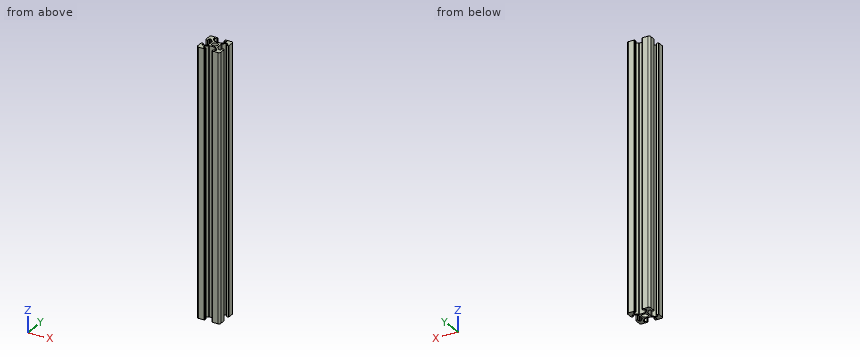
```python
from build123d import *

# Parameters (mm, degrees)
SKETCH_1_R      = 2.5
EXTRUDE_1_DEPTH = 230
FILLET_1_R      = 1.5


with BuildPart() as part:
    # 草图1 → 凸台-拉伸1 (new body)
    with BuildSketch(Plane.XY):
        with BuildLine():
            Line((20, 13.6), (20, 20))
            Line((20, 20), (13.6, 20))
            Line((13.6, 20), (13.6, 19.8))
            Line((13.6, 19.8), (13.2, 19.8))
            ThreePointArc((13.2, 19.8), (13.129289322, 19.770710678), (13.1, 19.7))
            Line((13.1, 19.7), (13.1, 18.3))
            ThreePointArc((13.1, 18.3), (13.129289322, 18.229289322), (13.2, 18.2))
            Line((13.2, 18.2), (15.2, 18.2))
            ThreePointArc((15.2, 18.2), (15.412132034, 18.112132034), (15.5, 17.9))
            Line((15.5, 17.9), (15.5, 16.974873734))
            ThreePointArc((15.5, 16.974873734), (15.423879533, 16.592190302), (15.207106781, 16.267766953))
            Line((15.207106781, 16.267766953), (13.132233047, 14.192893219))
            ThreePointArc((13.132233047, 14.192893219), (12.807809698, 13.976120467), (12.425126266, 13.9))
            Line((12.425126266, 13.9), (7.574873734, 13.9))
            ThreePointArc((7.574873734, 13.9), (7.192190302, 13.976120467), (6.867766953, 14.192893219))
            Line((6.867766953, 14.192893219), (4.792893219, 16.267766953))
            ThreePointArc((4.792893219, 16.267766953), (4.576120467, 16.592190302), (4.5, 16.974873734))
            Line((4.5, 16.974873734), (4.5, 17.9))
            ThreePointArc((4.5, 17.9), (4.587867966, 18.112132034), (4.8, 18.2))
            Line((4.8, 18.2), (6.8, 18.2))
            ThreePointArc((6.8, 18.2), (6.870710678, 18.229289322), (6.9, 18.3))
            Line((6.9, 18.3), (6.9, 19.7))
            ThreePointArc((6.9, 19.7), (6.870710678, 19.770710678), (6.8, 19.8))
            Line((6.8, 19.8), (6.4, 19.8))
            Line((6.4, 19.8), (6.4, 20))
            Line((6.4, 20), (0, 20))
            Line((0, 20), (0, 13.6))
            Line((0, 13.6), (0.2, 13.6))
            Line((0.2, 13.6), (0.2, 13.2))
            ThreePointArc((0.2, 13.2), (0.229289322, 13.129289322), (0.3, 13.1))
            Line((0.3, 13.1), (1.7, 13.1))
            ThreePointArc((1.7, 13.1), (1.770710678, 13.129289322), (1.8, 13.2))
            Line((1.8, 13.2), (1.8, 15.2))
            ThreePointArc((1.8, 15.2), (1.887867966, 15.412132034), (2.1, 15.5))
            Line((2.1, 15.5), (3.025126266, 15.5))
            ThreePointArc((3.025126266, 15.5), (3.407809698, 15.423879533), (3.732233047, 15.207106781))
            Line((3.732233047, 15.207106781), (5.807106781, 13.132233047))
            ThreePointArc((5.807106781, 13.132233047), (6.023879533, 12.807809698), (6.1, 12.425126266))
            Line((6.1, 12.425126266), (6.1, 7.574873734))
            ThreePointArc((6.1, 7.574873734), (6.023879533, 7.192190302), (5.807106781, 6.867766953))
            Line((5.807106781, 6.867766953), (3.732233047, 4.792893219))
            ThreePointArc((3.732233047, 4.792893219), (3.407809698, 4.576120467), (3.025126266, 4.5))
            Line((3.025126266, 4.5), (2.1, 4.5))
            ThreePointArc((2.1, 4.5), (1.887867966, 4.587867966), (1.8, 4.8))
            Line((1.8, 4.8), (1.8, 6.8))
            ThreePointArc((1.8, 6.8), (1.770710678, 6.870710678), (1.7, 6.9))
            Line((1.7, 6.9), (0.3, 6.9))
            ThreePointArc((0.3, 6.9), (0.229289322, 6.870710678), (0.2, 6.8))
            Line((0.2, 6.8), (0.2, 6.4))
            Line((0.2, 6.4), (0, 6.4))
            Line((0, 6.4), (0, 0))
            Line((0, 0), (6.4, 0))
            Line((6.4, 0), (6.4, 0.2))
            Line((6.4, 0.2), (6.8, 0.2))
            ThreePointArc((6.8, 0.2), (6.870710678, 0.229289322), (6.9, 0.3))
            Line((6.9, 0.3), (6.9, 1.7))
            ThreePointArc((6.9, 1.7), (6.870710678, 1.770710678), (6.8, 1.8))
            Line((6.8, 1.8), (4.8, 1.8))
            ThreePointArc((4.8, 1.8), (4.587867966, 1.887867966), (4.5, 2.1))
            Line((4.5, 2.1), (4.5, 3.025126266))
            ThreePointArc((4.5, 3.025126266), (4.576120467, 3.407809698), (4.792893219, 3.732233047))
            Line((4.792893219, 3.732233047), (6.867766953, 5.807106781))
            ThreePointArc((6.867766953, 5.807106781), (7.192190302, 6.023879533), (7.574873734, 6.1))
            Line((7.574873734, 6.1), (12.425126266, 6.1))
            ThreePointArc((12.425126266, 6.1), (12.807809698, 6.023879533), (13.132233047, 5.807106781))
            Line((13.132233047, 5.807106781), (15.207106781, 3.732233047))
            ThreePointArc((15.207106781, 3.732233047), (15.423879533, 3.407809698), (15.5, 3.025126266))
            Line((15.5, 3.025126266), (15.5, 2.1))
            ThreePointArc((15.5, 2.1), (15.412132034, 1.887867966), (15.2, 1.8))
            Line((15.2, 1.8), (13.2, 1.8))
            ThreePointArc((13.2, 1.8), (13.129289322, 1.770710678), (13.1, 1.7))
            Line((13.1, 1.7), (13.1, 0.3))
            ThreePointArc((13.1, 0.3), (13.129289322, 0.229289322), (13.2, 0.2))
            Line((13.2, 0.2), (13.6, 0.2))
            Line((13.6, 0.2), (13.6, 0))
            Line((13.6, 0), (20, 0))
            Line((20, 0), (20, 6.4))
            Line((20, 6.4), (19.8, 6.4))
            Line((19.8, 6.4), (19.8, 6.8))
            ThreePointArc((19.8, 6.8), (19.770710678, 6.870710678), (19.7, 6.9))
            Line((19.7, 6.9), (18.3, 6.9))
            ThreePointArc((18.3, 6.9), (18.229289322, 6.870710678), (18.2, 6.8))
            Line((18.2, 6.8), (18.2, 4.8))
            ThreePointArc((18.2, 4.8), (18.112132034, 4.587867966), (17.9, 4.5))
            Line((17.9, 4.5), (16.974873734, 4.5))
            ThreePointArc((16.974873734, 4.5), (16.592190302, 4.576120467), (16.267766953, 4.792893219))
            Line((16.267766953, 4.792893219), (14.192893219, 6.867766953))
            ThreePointArc((14.192893219, 6.867766953), (13.976120467, 7.192190302), (13.9, 7.574873734))
            Line((13.9, 7.574873734), (13.9, 12.425126266))
            ThreePointArc((13.9, 12.425126266), (13.976120467, 12.807809698), (14.192893219, 13.132233047))
            Line((14.192893219, 13.132233047), (16.267766953, 15.207106781))
            ThreePointArc((16.267766953, 15.207106781), (16.592190302, 15.423879533), (16.974873734, 15.5))
            Line((16.974873734, 15.5), (17.9, 15.5))
            ThreePointArc((17.9, 15.5), (18.112132034, 15.412132034), (18.2, 15.2))
            Line((18.2, 15.2), (18.2, 13.2))
            ThreePointArc((18.2, 13.2), (18.229289322, 13.129289322), (18.3, 13.1))
            Line((18.3, 13.1), (19.7, 13.1))
            ThreePointArc((19.7, 13.1), (19.770710678, 13.129289322), (19.8, 13.2))
            Line((19.8, 13.2), (19.8, 13.6))
            Line((19.8, 13.6), (20, 13.6))
        make_face()
        with Locations((10, 10)):
            Circle(SKETCH_1_R, mode=Mode.SUBTRACT)
    extrude(amount=EXTRUDE_1_DEPTH)

    # 圆角1
    fillet_1_edges = [part.edges().sort_by_distance(p)[0] for p in [
        (0, 0, 115),
        (0, 20, 115),
        (20, 20, 115),
        (20, 0, 115),
    ]]
    fillet(fillet_1_edges, radius=FILLET_1_R)


solid = part.part
```
The listing builds one solid part. Answer for the finished solid, in the listing's coordinates (mm). Round coordinates to 2 decimals unless told otherwise and drop trailing zeros. Order: outer loops, then holes, each group sorted by start corner. A loop starts at its lowest first (then second) coordinate and runs counter-clockwise, first axis right, second up. Notation, with made-up numbers: (54.5, 3) -> (111.5, 3) arc R19 ccw to (111.5, 19) -> close; hole circle Ø3 at (-11.5, 7). An arc over 180 degrees is marked (long way). Answer as CSV lines item,"result". Start each with the question number.
(1) Flat-ended cylindrical pins translate along their axes: pin 1 Ø4.5 at (x, y) = (10, 10) entering from +Z (3 decimals); pin 2 Ø1.5 at (y, z) = (11, 31.5) entering from +X; pin 3 Ø2.5 at (x, z) = (10, 152) entering from -Y; pin 4 Ø5.5 at (x, z) = (10, 62) entering from +Y. Find the tip coordinate at first contact, or state that the pin passes through.
(2) Find the intervals of material crossed by probe 1 along Y at (x, z) = (4.75, 175); probe 2 along X at (y, z) = (2.5, 200); probe 3 along Y at (x, z) = (10, 168), in increasing order. Write a range as from..to.
(3) The part is cut by section A-A (y = 10). Determine the outline of the cut face in (x, z).
Evaluation:
1,pin 1,"through"
1,pin 2,"x = 13.9"
1,pin 3,"y = 6.1"
1,pin 4,"y = 13.95"
2,probe 1,"0..1.8, 3.69..5.81, 14.19..16.31, 18.2..20"
2,probe 2,"0..4.5, 15.5..20"
2,probe 3,"6.1..7.5, 12.5..13.9"
3,outline,"(6.1, 0) -> (7.5, 0) -> (7.5, 230) -> (6.1, 230) -> close; (12.5, 0) -> (13.9, 0) -> (13.9, 230) -> (12.5, 230) -> close"
